```python
from build123d import *

# Parameters (mm, degrees)
EXTRUDE_1_DEPTH     = 5
EXTRUDE_2_DEPTH     = 5
SKETCH_3_R          = 1.75
CUT_EXTRUDE_1_DEPTH = 21
SKETCH_4_R          = 1.75
CUT_EXTRUDE_2_DEPTH = 21
FILLET_1_R          = 5
FILLET_2_R          = 10
SKETCH_6_R          = 1.5
CUT_EXTRUDE_4_DEPTH = 10
SKETCH_7_R          = 7.5
CUT_EXTRUDE_5_DEPTH = 10
SKETCH_8_R          = 12.5
CUT_EXTRUDE_6_DEPTH = 10


with BuildPart() as part:
    # 草图1 → 凸台-拉伸1 (new body)
    with BuildSketch(Plane(origin=(0, 0, 0), x_dir=(1, 0, 0), z_dir=(0, 1, 0))):
        with BuildLine():
            ThreePointArc((0, 24), (-24, 0), (0, -24))
            Line((0, -24), (60, -24))
            Line((60, -24), (60, 24))
            Line((60, 24), (0, 24))
        make_face()
    extrude(amount=EXTRUDE_1_DEPTH)

    # 草图2 → 凸台-拉伸2 (add)
    with BuildSketch(Plane(origin=(60, 0, 0), x_dir=(0, 0, -1), z_dir=(1, 0, 0))):
        with BuildLine():
            ThreePointArc((24, 40), (0, 64), (-24, 40))
            Line((-24, 40), (-24, 0))
            Line((-24, 0), (24, 0))
            Line((24, 0), (24, 40))
        make_face()
    extrude(amount=-EXTRUDE_2_DEPTH)

    # 草图3 → 切除-拉伸1 (cut)
    with BuildSketch(Plane(origin=(0, 5, 0), x_dir=(1, 0, 0), z_dir=(0, 1, 0))):
        with Locations(Location((-13.5, 0, 0), (0, 0, 270))):
            Circle(SKETCH_3_R)
        with Locations(Location((-6.75, 11.691342951, 0), (0, 0, 270))):
            Circle(SKETCH_3_R)
        with Locations(Location((6.75, 11.691342951, 0), (0, 0, 270))):
            Circle(SKETCH_3_R)
        with Locations(Location((13.5, 0, 0), (0, 0, 270))):
            Circle(SKETCH_3_R)
        with Locations(Location((6.75, -11.691342951, 0), (0, 0, 270))):
            Circle(SKETCH_3_R)
        with Locations(Location((-6.75, -11.691342951, 0), (0, 0, 270))):
            Circle(SKETCH_3_R)
    extrude(amount=-CUT_EXTRUDE_1_DEPTH, mode=Mode.SUBTRACT)

    # 草图4 → 切除-拉伸2 (cut)
    with BuildSketch(Plane(origin=(60, 0, 0), x_dir=(0, 0, -1), z_dir=(1, 0, 0))):
        with Locations((-13.435028843, 53.435028843)):
            Circle(SKETCH_4_R)
        with Locations((13.435028843, 53.435028843)):
            Circle(SKETCH_4_R)
        with Locations((13.435028843, 26.564971157)):
            Circle(SKETCH_4_R)
        with Locations((-13.435028843, 26.564971157)):
            Circle(SKETCH_4_R)
    extrude(amount=-CUT_EXTRUDE_2_DEPTH, mode=Mode.SUBTRACT)

    # 圆角1
    fillet_1_edges = [part.edges().sort_by_distance(p)[0] for p in [
        (55, 5, 0),
    ]]
    fillet(fillet_1_edges, radius=FILLET_1_R)

    # 圆角2
    fillet_2_edges = [part.edges().sort_by_distance(p)[0] for p in [
        (60, 0, 0),
    ]]
    fillet(fillet_2_edges, radius=FILLET_2_R)

    # 草图6 → 切除-拉伸4 (cut)
    with BuildSketch(Plane(origin=(0, 5, 0), x_dir=(1, 0, 0), z_dir=(0, 1, 0))):
        with Locations(Location((0, 20, 0), (0, 0, 270))):
            Circle(SKETCH_6_R)
        with Locations(Location((35, 20, 0), (0, 0, 270))):
            Circle(SKETCH_6_R)
        with Locations(Location((35, -20, 0), (0, 0, 270))):
            Circle(SKETCH_6_R)
        with Locations(Location((0, -20, 0), (0, 0, 270))):
            Circle(SKETCH_6_R)
        with Locations(Location((-20, 0, 0), (0, 0, 270))):
            Circle(SKETCH_6_R)
    extrude(amount=-CUT_EXTRUDE_4_DEPTH, mode=Mode.SUBTRACT)

    # 草图7 → 切除-拉伸5 (cut)
    with BuildSketch(Plane(origin=(0, 5, 0), x_dir=(1, 0, 0), z_dir=(0, 1, 0))):
        with Locations(Location((0, 0, 0), (0, 0, 270))):
            Circle(SKETCH_7_R)
    extrude(amount=-CUT_EXTRUDE_5_DEPTH, mode=Mode.SUBTRACT)

    # 草图8 → 切除-拉伸6 (cut)
    with BuildSketch(Plane(origin=(60, 0, 0), x_dir=(0, 0, -1), z_dir=(1, 0, 0))):
        with Locations((0, 40)):
            Circle(SKETCH_8_R)
    extrude(amount=-CUT_EXTRUDE_6_DEPTH, mode=Mode.SUBTRACT)


solid = part.part
```
Verification items for the finished model (mm, model axes). Give positions to 0.01 mm unless a question says otherwise; leave off trailing zeros. Order: outer loops, then holes, each group sorted by start corner. A loop starts at its lowest first (then second) coordinate and runs counter-clockwise, first axis right, second up. Notation, with made-up numbers: M 16,-16.75 L 39,-16.75 A35 cw 39,15.25 Z; hole C 30,-8.5 d6. An arc over 180 degrees is marked long. Return JSON: item names as keys, results as strings. Group by question number.
1) Scan lines: line 1 (X direction, y = 2, z = -20); line 2 (X direction, y = 2.25, z = 0); line 3 (X direction, y = 3.35, z = 20). Record each from-to range of solid material in increasing order.
2) Section check A-A on y = 46. Record the cut outline in (x, z).
3) Go/stop test with flat-tipped pins: pin 1 Ø24 at (x, z) = (20, 4) entering from +Y; pin 2 Ø1.8 at (x, z) = (0, 20) entering from +Y; pin 3 Ø24 at (y, z) = (35, -10) entering from -X. Record where each tip stops, or that it passes through.
4) Mould release check, pull along Z, two halves, no side actions. Record for faces 1 (the face through (15.235, 2.535, -0.228)), 2 (the face through (-23.994, 2.465, -0.528)), 3 (the face through (56.99, 2.85, -0.34)): pulls with the +Z half, pulls with the -Z half, needs draft (parallel to the pull), parting line crosses it, or undercut.
5) Section check B-B on x = 35. Record the cut outline in (y, z), and give its area (3 significant figures).
6) Section check C-C on z = 9. Record the cut outline in (x, y), and give its area (3 significant figures).
7) Section check D-D on z = -20. Record the cut outline in (x, y).
Answer block:
{
 "1": {"line 1": "x = -13.27 to -1.5, 1.5 to 33.5, 36.5 to 56", "line 2": "x = -24 to -21.5, -18.5 to -15.25, -11.75 to -7.5, 7.5 to 11.75, 15.25 to 56.32", "line 3": "x = -13.27 to -1.5, 1.5 to 33.5, 36.5 to 57.47"},
 "2": {"outline": "M 55,-23.24 L 60,-23.24 L 60,-10.97 L 55,-10.97 Z; M 55,10.97 L 60,10.97 L 60,23.24 L 55,23.24 Z"},
 "3": {"pin 1": "stops at y = 5", "pin 2": "passes through", "pin 3": "stops at x = 55"},
 "4": {"face 1": "undercut", "face 2": "parting line crosses it", "face 3": "needs draft"},
 "5": {"outline": "M 0,-24 L 5,-24 L 5,-21.5 L 0,-21.5 Z; M 0,-18.5 L 5,-18.5 L 5,18.5 L 0,18.5 Z; M 0,21.5 L 5,21.5 L 5,24 L 0,24 Z", "area": "210 mm^2"},
 "6": {"outline": "M -22.25,0 L 50,0 A10 ccw 60,10 L 60,31.33 L 55,31.33 L 55,10 A5 cw 50,5 L -22.25,5 Z; M 55,48.67 L 60,48.67 L 60,62.25 L 55,62.25 Z", "area": "595 mm^2"},
 "7": {"outline": "M -13.27,0 L -1.5,0 L -1.5,5 L -13.27,5 Z; M 1.5,0 L 33.5,0 L 33.5,5 L 1.5,5 Z; M 36.5,0 L 50,0 A10 ccw 60,10 L 60,53.27 L 55,53.27 L 55,10 A5 cw 50,5 L 36.5,5 Z"}
}
